The model under review builds one solid part; all positions refer to its coordinate system, in mm. A direction names the side the tool comes from. Round coordinates to 2 decimals unless told otherwise and drop trailing zeros. Order: outer loops, then holes, each group sorted by start corner. A loop starts at its lowest first (then second) coordinate and runs counter-clockwise, first axis right, second up. Notation, with made-up numbers: M 16,19.5 L 27,19.5 A27 ccw 27,42.5 Z; hole C -0.5,-37 d1. An arc over 180 degrees is marked long. Answer as CSV lines item,"result". Start each with the question number.
from build123d import *

# Parameters (mm, degrees)
SKETCH1_R           = 1.4224
SKETCH1_R_2         = 1.524
BOSS_EXTRUDE1_DEPTH = 3.175


with BuildPart() as part:
    # Sketch1 → Boss-Extrude1 (new body)
    with BuildSketch(Plane.XY):
        with BuildLine():
            Line((-70.6755, 6.936048929), (-1.801090909, 15.133197664))
            ThreePointArc((-1.801090909, 15.133197664), (15.24, 0), (-1.801090909, -15.133197664))
            Line((-1.801090909, -15.133197664), (-70.6755, -6.936048929))
            ThreePointArc((-70.6755, -6.936048929), (-76.835, 0), (-70.6755, 6.936048929))
        make_face()
        with Locations((-69.85, 0)):
            Circle(SKETCH1_R, mode=Mode.SUBTRACT)
        with Locations((7.184204897, -7.184204897)):
            Circle(SKETCH1_R_2, mode=Mode.SUBTRACT)
        with Locations((-9.813806395, -2.629601498)):
            Circle(SKETCH1_R_2, mode=Mode.SUBTRACT)
        with Locations((2.629601498, 9.813806395)):
            Circle(SKETCH1_R_2, mode=Mode.SUBTRACT)
        with BuildLine():
            Line((-0.25049165, 3.992149037), (-3.992149037, 0.25049165))
            ThreePointArc((-3.992149037, 0.25049165), (2.828427125, -2.828427125), (-0.25049165, 3.992149037))
        make_face(mode=Mode.SUBTRACT)
    extrude(amount=BOSS_EXTRUDE1_DEPTH)


solid = part.part
Item 1: Wall thickness on probe 1 along X at (y, z) = (-3.5, 1); probe 2 along X at (y, z) = (-1, 2.75); probe 3 along Y at (x, z) = (2, 0.3): over which ranges is each line inside the solid? List them lowest first. Write a range as [from, to].
Item 2: Consider section B-B (z = 2.35). State how many separate pieces and enclosed holes the cut face has, and give its area (3 significant figures).
Item 3: Consider section D-D (y = -11.5). State the section outline as (x, z) points (3 decimals).
Item 4: The part is to be moulded in two halves that separate along Y. For faces 3 (the flat face through (-36.72, 10.977, 1.565)), 4 (the cylindrical face through (6.986, -5.673, 1.565)), 5 (the flat face through (-30, 0, 3.175)), 6 (the cylindrical face through (15.236, 0.36, 1.565)), say which applies: +Y half, -Y half, draft (parallel to the pull), parting line (faces both ways), or undercut.
Item 5: For pin 1 (2.5 mm diameter, centred on x = 2.63, y = 9.81, fed in from +Z); pin 2 (4 mm diameter, centred on x = -9.81, y = -2.63, fed in from +Z) (3 decimals), all flat-tipped, find the tip position at first contact; note any pin that passes through.
Item 6: Tool access review of faces 1 (the cylindrical face through (-76.834, -0.142, 1.565)), 2 (the flat face through (-2.095, 2.148, 1.565)): name each direction out of +Z, -Z, +X, -X, +Y, -Y from which nothing blocks a thin tool from reaching the whole face with its end or side.
Item 7: Consider section A-A (x = -69.85). State the section outline as (y, z) points (3 decimals), and give its area (3 significant figures).
Item 8: Consider section C-C (x = -56). State the section outline as (y, z) points (3 decimals), and give its area (3 significant figures).
Reported:
1,probe 1,"x = [-75.89, -11.06], [-8.56, -1.94], [1.94, 14.83]"
1,probe 2,"x = [-76.76, -70.86], [-68.84, -3.87], [3.87, 15.21]"
1,probe 3,"y = [-15.11, -3.46], [3.46, 8.43], [11.2, 15.11]"
2,separate pieces,"1"
2,enclosed holes,"5"
2,area,"1,930 mm²"
3,outline,"M -32.328,0 L 10,0 L 10,3.175 L -32.328,3.175 Z"
4,face 3,"+Y half"
4,face 4,"undercut"
4,face 5,"draft"
4,face 6,"parting line"
5,pin 1,"passes through"
5,pin 2,"stops at z = 3.175"
6,face 1,"+Z, -Z, -X"
6,face 2,"+Z, -Z"
7,outline,"M -7.034,0 L -1.422,0 L -1.422,3.175 L -7.034,3.175 Z; M 1.422,0 L 7.034,0 L 7.034,3.175 L 1.422,3.175 Z"
7,area,"35.6 mm²"
8,outline,"M -8.683,0 L 8.683,0 L 8.683,3.175 L -8.683,3.175 Z"
8,area,"55.1 mm²"
